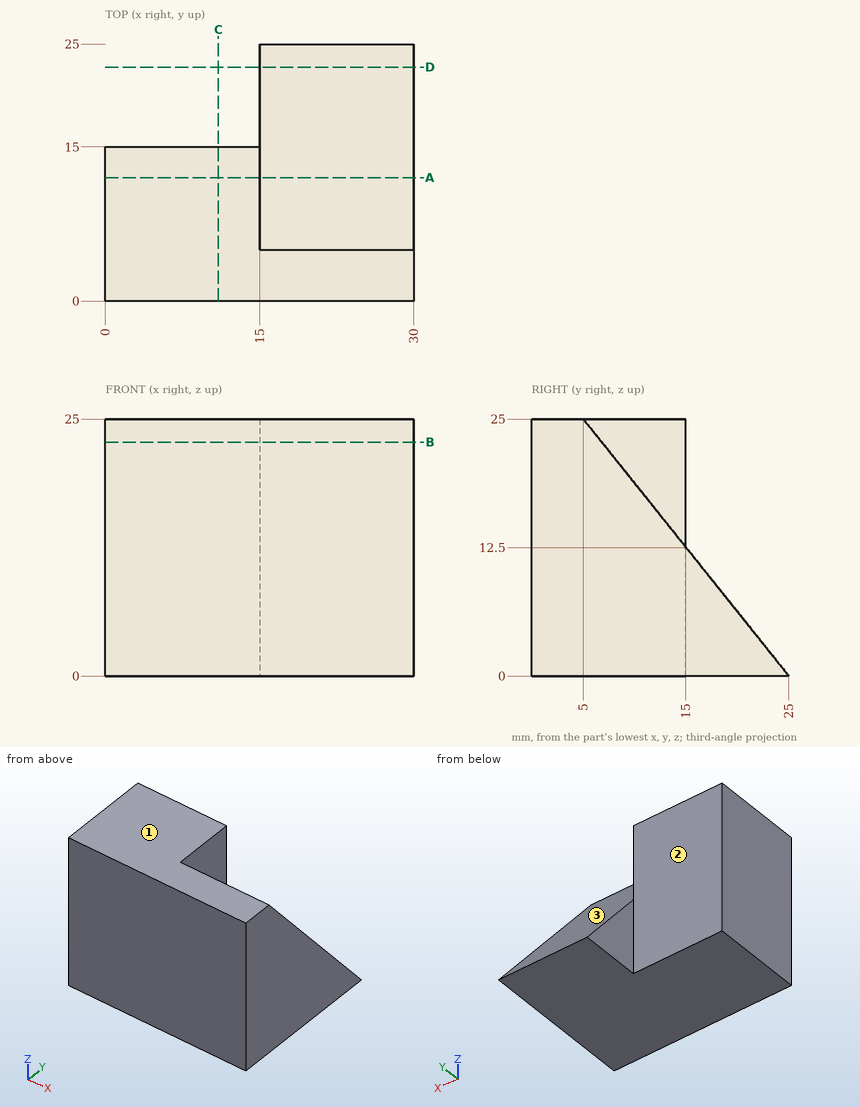
Design review of the part shown in the three views and the two pictorial views. Dimensions are in mm from the part's minimum x, y and z. A direction names the side the tool comes from. Give positions to 0.01 mm unless a question says otherwise; leave off trailing zeros. Write each loop counter-clockwise with the first axis right and the second up, starting at its lowest first coordinate (ties: lowest second). Pieces come first, ordered by that corner, then holes.
(1) Add section C-C (x = 11). Give the boundary of the cut face in (y, z), and give its area (3 significant figures).
Checked values:
outline: (0, 0) - (15, 0) - (15, 25) - (0, 25) - close
area: 375 mm2
(2) Wall thickness on line 1 along Y through (x, z) = (7, 17.5): over which ranges is the line inside the solid? List them lowest first.
Checked values:
line 1: y = 0 to 15
(3) Add section B-B (z = 22.75). Give the boundary of the cut face in (x, y), and give its area (3 significant figures).
Checked values:
outline: (0, 0) - (30, 0) - (30, 6.8) - (15, 6.8) - (15, 15) - (0, 15) - close
area: 327 mm2
(4) Add section D-D (y = 22.75). Give the boundary of the cut face in (x, z), and give its area (3 significant figures).
Checked values:
outline: (15, 0) - (30, 0) - (30, 2.81) - (15, 2.81) - close
area: 42.2 mm2
(5) Tool access review of the marked faces 1, 2 and 3: name each direction out of +Z, -Z, +X, -X, +Y, -Y from which nothing blocks a thin tool from reaching the whole face with its end or side.
Checked values:
face 1: +Z, +X, -X, +Y, -Y
face 2: +Z, -Z, -X, +Y
face 3: +Z, +X, +Y
(6) Clearance check with flat-ended pins moving along their axes: pin 1 Ø4 at (x, z) = (9.5, 6.5) entering from -Y; pin 2 Ø1.5 at (x, z) = (16, 16) entering from +Y; pin 3 Ø7.5 at (x, z) = (9.5, 14) entering from +Y; pin 4 Ø8 at (y, z) = (19.5, 7.5) entering from -X. State where each tip first meets the part, or that it passes through.
Checked values:
pin 1: stops at y = 0
pin 2: stops at y = 12.8
pin 3: stops at y = 15
pin 4: stops at x = 15
(7) Add section A-A (y = 12). Give the boundary of the cut face in (x, z), and give its area (3 significant figures).
Checked values:
outline: (0, 0) - (30, 0) - (30, 16.25) - (15, 16.25) - (15, 25) - (0, 25) - close
area: 619 mm2
